Check sheet for the modelled part. Datum: model origin and axes. Units: mm. Coordinates: 2 decimals unless noted, no trailing zeros. Loops run counter-clockwise (first coordinate to the right, second up) from the corner with the lowest first, then second, coordinate; pieces in that order, holes last. Notation, with made-up numbers: (51, 76) -> (73, 76) arc R19 ccw to (73, 106) -> close; hole circle Ø1 at (21, -8.5). An arc over 180 degrees is marked (long way). Use one line per item in the form item = value.
from build123d import *

# Parameters (mm, degrees)
F1_DEPTH = 3
F3_DEPTH = 25.4
F4_W     = 9.96188
F4_H     = 735.775
F5_DEPTH = 25.4


with BuildPart() as f1:
    # F0 (on Front) → F1 (new body)
    with BuildSketch(Plane.XZ):
        Polygon((-76.2, 698.5), (-280.5938, 698.5), (-280.5938, -41.275), (280.59888, -41.275), (280.59888, 698.5), (76.2, 698.5), (76.2, 0), (0, 0), (-76.2, 0), align=None)
    extrude(amount=F1_DEPTH)

    # F2 (on face) → F3 (cut)
    with BuildSketch(Plane.XZ.offset(3)):
        Polygon((-280.5938, -37.275), (-280.5938, -41.275), (-280.2390158176, -41.275), (280.59888, -41.275), (280.59888, -37.275), align=None)
    extrude(amount=-F3_DEPTH, mode=Mode.SUBTRACT)

    # F4 (on face) → F5 (cut)
    with BuildSketch(Plane.XZ.offset(3)):
        with Locations((275.61794, 330.6125)):
            Rectangle(F4_W, F4_H)
    extrude(amount=-F5_DEPTH, mode=Mode.SUBTRACT)


solid = f1.part
(1) Scan lines: line 1 along X through (y, z) = (-2.75, 515.5); line 2 along Z through (x, y) = (13, -1.65) (3 decimals). Record each from-to range of solid material in increasing order.
Established:
line_1 = -280.59 to -76.2, 76.2 to 270.64
line_2 = -37.275 to 0
(2) Section check B-B, the plane y = -1.6. Record the boundary of the cut face in (x, z) (3 decimals), plus the area to 3 significant figures.
Established:
outline = (-280.594, -37.275) -> (270.637, -37.275) -> (270.637, 698.5) -> (76.2, 698.5) -> (76.2, 0) -> (-76.2, 0) -> (-76.2, 698.5) -> (-280.594, 698.5) -> close
area = 299,000 mm²
(3) Go/stop test with flat-tipped pins: P1, Ø1.5, axis at x = 25.5, y = -2, coming from the +Z side; P2, Ø2, axis at x = 173.5, z = 625, coming from the +Y side. Record where each tip stops, or that it passes through.
Established:
P1 = 0
P2 = 0
(4) Section check A-A, the plane z = 216.5. Record the boundary of the cut face in (x, y).
Established:
outline = (-280.59, -3) -> (-76.2, -3) -> (-76.2, 0) -> (-280.59, 0) -> close; (76.2, -3) -> (270.64, -3) -> (270.64, 0) -> (76.2, 0) -> close
(5) Section check C-C, the plane x = 11.5. Record the boundary of the cut face in (y, z) (3 decimals), plus the area to 3 significant figures.
Established:
outline = (-3, -37.275) -> (0, -37.275) -> (0, 0) -> (-3, 0) -> close
area = 112 mm²
